Here's how the part is built. I have some questions about the finished solid (model axes, mm). Face numbers are marked on the shaded views. A direction names the side the tool comes from. Round coordinates to 2 decimals unless told otherwise and drop trailing zeros. Loops run counter-clockwise (first coordinate to the right, second up) from the corner with the lowest first, then second, coordinate; pieces in that order, holes last. Notation, with made-up numbers: (53.25, 25.5) - (109.25, 25.5) arc R29 ccw to (109.25, 59.5) - close; hole circle Ø4 at (-13, 35). An arc over 180 degrees is marked (long way). Answer as a JSON object with one key per item and string values. Group by question number.
1) If we mould it in two halves opening along Z, with no side actions, what happens to the marked faces 1, 2 and 3? For each: pulls with the +Z half, pulls with the -Z half, needs draft (parallel to the pull), parting line crosses it, or undercut.
2) I want a section at A-A, the plane y = -25. Please give me the cut outline in (x, z).
3) I want a section at C-C, the plane y = -48. Give the number of separate pieces and of enclosed holes in the cut face, then the cut area to 3 significant figures.
4) I want a section at B-B, the plane y = 8. Please give me the cut outline in (x, z).
5) Will these pins go through, and if not, where does the flat tip stop? P1, Ø3, axis at x = 3.5, z = -3, coming from the +Y side; P2, Ø6, axis at x = -7, y = -17, coming from the -Z side; P3, Ø7, axis at x = -20, z = -10, coming from the -Y side; P4, Ø3.5, axis at x = -2.5, y = 8, coming from the +Z side.
6) Which directions (+Z, -Z, +X, -X, +Y, -Y) give clear straight access to the entire face, cutting with the end or side of a thin tool? Please do the marked faces 4, 5 and 6.
7) If I drill on line 1 along Y through (x, z) = (-2.5, 1.9); line 2 along X through (y, z) = (12, -10); line 3 along Y through (x, z) = (23, 1.95), over which ranges is the centre line in solid material (lowest first)? Write a range as [from, to].
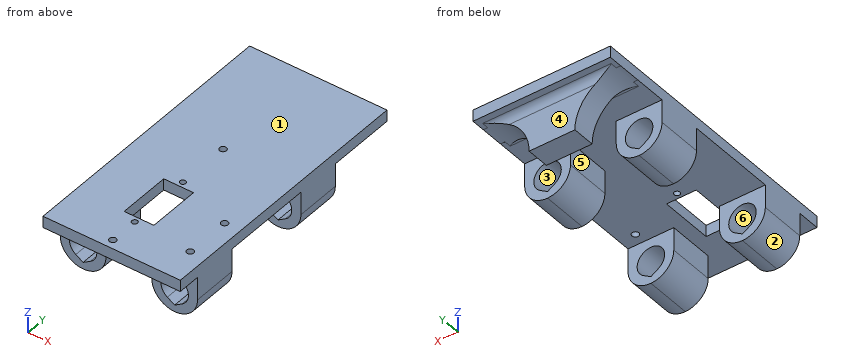
from build123d import *

# Parameters (mm, degrees)
SKETCH1_W           = 60
SKETCH1_H           = 120
SKETCH1_R           = 1.5
SKETCH1_R_2         = 1.25
SKETCH1_W_2         = 13
SKETCH1_H_2         = 23
BOSS_EXTRUDE1_DEPTH = 5
SKETCH2_W           = 20
SKETCH2_H           = 20
BOSS_EXTRUDE2_DEPTH = 20
CUT_EXTRUDE1_DEPTH  = 116.758369028
FILLET1_R           = 10
SKETCH4_W           = 60
SKETCH4_H           = 10
BOSS_EXTRUDE3_DEPTH = 19
CUT_EXTRUDE2_DEPTH  = 10
FILLET2_R           = 3


with BuildPart() as part:
    # Sketch1 → Boss-Extrude1 (new body)
    with BuildSketch(Plane.XY):
        Rectangle(SKETCH1_W, SKETCH1_H)
        with Locations((23, -25)):
            Circle(SKETCH1_R, mode=Mode.SUBTRACT)
        with Locations((23, -45)):
            Circle(SKETCH1_R, mode=Mode.SUBTRACT)
        with Locations((-2.5, -56)):
            Circle(SKETCH1_R, mode=Mode.SUBTRACT)
        with Locations((-2.5, 8)):
            Circle(SKETCH1_R, mode=Mode.SUBTRACT)
        with Locations((-2.5, -15.3)):
            Circle(SKETCH1_R_2, mode=Mode.SUBTRACT)
        with Locations((-2.5, -43.3)):
            Circle(SKETCH1_R_2, mode=Mode.SUBTRACT)
        with Locations((-2.5, -29.3)):
            Rectangle(SKETCH1_W_2, SKETCH1_H_2, mode=Mode.SUBTRACT)
    extrude(amount=BOSS_EXTRUDE1_DEPTH)

    # Sketch2 → Boss-Extrude2 (add)
    with BuildSketch(Plane(origin=(0, 0, 0), x_dir=(-1, 0, 0), z_dir=(0, 0, -1))):
        with Locations((-20, -40)):
            Rectangle(SKETCH2_W, SKETCH2_H)
        with Locations((20, -40)):
            Rectangle(SKETCH2_W, SKETCH2_H)
        with Locations((20, 20)):
            Rectangle(SKETCH2_W, SKETCH2_H)
        with Locations((-20, 20)):
            Rectangle(SKETCH2_W, SKETCH2_H)
    extrude(amount=BOSS_EXTRUDE2_DEPTH)

    # Sketch3 → Cut-Extrude1 (cut, through all)
    with BuildSketch(Plane.XZ.offset(50)):
        with BuildLine():
            Line((-23.188342055, -15.08276253), (-20, -17.08276253))
            Line((-20, -17.08276253), (-16.811657945, -15.08276253))
            ThreePointArc((-16.811657945, -15.08276253), (-20, -4), (-23.188342055, -15.08276253))
        make_face()
        with BuildLine():
            Line((20, -17.08276253), (16.811657945, -15.08276253))
            ThreePointArc((16.811657945, -15.08276253), (20, -4), (23.188342055, -15.08276253))
            Line((23.188342055, -15.08276253), (20, -17.08276253))
        make_face()
    extrude(amount=-CUT_EXTRUDE1_DEPTH, mode=Mode.SUBTRACT)

    # Fillet1
    fillet1_edges = [part.edges().sort_by_distance(p)[0] for p in [
        (-10, -40, -20),
        (-30, -40, -20),
        (-30, 20, -20),
        (-10, 20, -20),
        (30, 20, -20),
        (10, 20, -20),
        (10, -40, -20),
        (30, -40, -20),
    ]]
    fillet(fillet1_edges, radius=FILLET1_R - 0.0001)  # a hair under: the kernel refuses the full size

    # Sketch4 → Boss-Extrude3 (add)
    with BuildSketch(Plane(origin=(0, 0, 0), x_dir=(-1, 0, 0), z_dir=(0, 0, -1))):
        with Locations((0, 49)):
            Rectangle(SKETCH4_W, SKETCH4_H)
    extrude(amount=BOSS_EXTRUDE3_DEPTH)

    # Sketch5 → Cut-Extrude2 (cut)
    with BuildSketch(Plane(origin=(0, 54, 0), x_dir=(1, 0, 0), z_dir=(0, 1, 0))):
        with BuildLine():
            Line((-10, 19), (-30, 19))
            Line((-30, 19), (-30, 0))
            ThreePointArc((-30, 0), (-15.921541487, 5.206885776), (-10, 19))
        make_face()
        with BuildLine():
            Line((10, 19), (30, 19))
            Line((30, 19), (30, 0))
            ThreePointArc((30, 0), (15.921541487, 5.206885776), (10, 19))
        make_face()
    extrude(amount=-CUT_EXTRUDE2_DEPTH, mode=Mode.SUBTRACT)

    # Fillet2
    fillet2_edges = [part.edges().sort_by_distance(p)[0] for p in [
        (0, 44, 0),
        (0, 54, 0),
    ]]
    fillet(fillet2_edges, radius=FILLET2_R)


solid = part.part
Outcome:
{
 "1": {"face 1": "pulls with the +Z half", "face 2": "pulls with the -Z half", "face 3": "undercut"},
 "2": {"outline": "(-30, 0) - (-9, 0) - (-9, 5) - (-30, 5) - close; (4, 0) - (21.5, 0) - (21.5, 5) - (4, 5) - close; (24.5, 0) - (30, 0) - (30, 5) - (24.5, 5) - close"},
 "3": {"separate pieces": "1", "enclosed holes": "2", "area": "783 mm^2"},
 "4": {"outline": "(-30, 0) - (-4, 0) - (-4, 5) - (-30, 5) - close; (-1, 0) - (30, 0) - (30, 5) - (-1, 5) - close"},
 "5": {"P1": "y = 54.4", "P2": "z = 0", "P3": "through", "P4": "z = 5"},
 "6": {"face 4": "-Z, +X, -X, +Y", "face 5": "-Z, -Y", "face 6": "+Y, -Y"},
 "7": {"line 1": "[-60, -57.5], [-54.5, -44.55], [-42.05, -40.8], [-17.8, -16.55], [-14.05, 6.5], [9.5, 60]", "line 2": "[-30, -26], [-14, -10], [10, 14], [26, 30]", "line 3": "[-60, -46.5], [-43.5, -26.5], [-23.5, 60]"}
}
